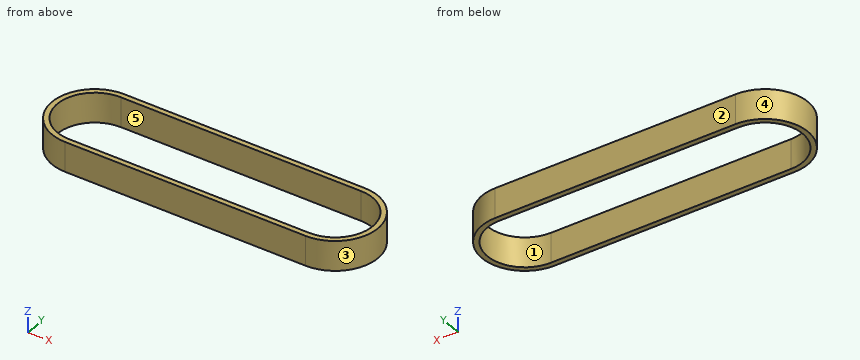
Autodesk Inventor part; units mm, degrees
ref_plane "YZ Plane" through (0, 0, 0) normal (1, 0, 0) x (0, 1, 0)
ref_plane "XZ Plane" through (0, 0, 0) normal (0, 1, 0) x (-1, 0, 0)
ref_plane "XY Plane" through (0, 0, 0) normal (0, 0, 1) x (1, 0, 0)
sketch "Sketch1" plane through (0, 0, 0) normal (0, 0, 1) x (1, 0, 0)
  arc A0 (0, -11.4595) -> (0, 11.4595) centre (0, 0) ccw construction
  arc A1 (-68.9989, 11.4595) -> (-68.9989, -11.4595) centre (-68.9989, 0) ccw construction
  line L0 (0, -11.4595) -> (-68.9989, -11.4595) construction
  line L1 (0, 11.4595) -> (-68.9989, 11.4595) construction
  dimension "Belt_Teeth" = 70
  dimension "Belt_Pitch2" = 3
  dimension "d0" = 22.919
  dimension "d1" = 22.919
  dimension "d2" = 36.0011
  dimension "d3" = 36.0011
  dimension "Center_Distance" = 68.9989
  dimension "d5" = 68.9989
sketch "Sketch2" plane through (0, 0, 0) normal (0, 0, 1) x (1, 0, 0)
  line L0 (35.7235, 34.2567) -> (38.7235, 34.2567)
  point P0 (0, 0)
  dimension "Belt_Pitch2" = 3
sketch "Sketch4" plane through (0, 0, 0) normal (0, 0, 1) x (1, 0, 0)
  line L0 (-16.1422, -21.869) -> (-14.1422, -21.869)
  line L1 (-16.1422, -21.869) -> (-16.1422, -20.349)
  arc A0 (-15.5872, -20.904) -> (-16.1422, -20.349) centre (-16.1422, -20.904) ccw
  line L2 (-15.5872, -20.904) -> (-15.5872, -20.959)
  arc A1 (-15.5872, -20.959) -> (-15.4372, -21.109) centre (-15.4372, -20.959) ccw
  line L3 (-15.4372, -21.109) -> (-14.8472, -21.109)
  line L4 (-14.1422, -21.869) -> (-14.1422, -20.349)
  arc A2 (-14.1422, -20.349) -> (-14.6972, -20.904) centre (-14.1422, -20.904) ccw
  arc A3 (-14.8472, -21.109) -> (-14.6972, -20.959) centre (-14.8472, -20.959) ccw
  line L5 (-14.6972, -20.959) -> (-14.6972, -20.904)
  line L6 (0, 11.4595) -> (-68.9989, 11.4595) construction
  arc A4 (-68.9989, 11.4595) -> (-68.9989, -11.4595) centre (-68.9989, 0) ccw construction
  line L7 (0, -11.4595) -> (-68.9989, -11.4595) construction
  arc A5 (0, -11.4595) -> (0, 11.4595) centre (0, 0) ccw construction
  arc A6 (-68.9989, 12.2195) -> (-68.9989, -12.2195) centre (-68.9989, 0) ccw
  line L8 (-68.9989, 12.2195) -> (0, 12.2195)
  arc A7 (0, -12.2195) -> (0, 12.2195) centre (0, 0) ccw
  line L9 (0, -12.2195) -> (-68.9989, -12.2195)
  arc A8 (-68.9989, 10.6995) -> (-68.9989, -10.6995) centre (-68.9989, 0) ccw
  line L10 (-68.9989, 10.6995) -> (0, 10.6995)
  arc A9 (0, -10.6995) -> (0, 10.6995) centre (0, 0) ccw
  line L11 (0, -10.6995) -> (-68.9989, -10.6995)
  point P0 (-15.1422, -21.109)
  point P1 (-15.1422, -21.869)
  dimension "d9" = 2
  dimension "d10" = 1.52
  dimension "d11" = 0.76
  dimension "d12" = 0.555
  dimension "d13" = 0.555
  dimension "d14" = 0.15
  dimension "d15" = 0.15
  dimension "belt_thickness" = 1.52
  dimension "d44" = 0.76
extrude "Extrusion2" add sketch "Sketch4" along normal mid plane 8.5 contours L8 A7 L9 A6
sketch "Sketch5" plane through (0, 0, 4.25) normal (0, 0, 1) x (1, 0, 0)
  line L0 (-68.9989, 10.6995) -> (0, 10.6995) construction
  arc A0 (0, -10.6995) -> (0, 10.6995) centre (0, 0) ccw construction
  line L1 (0, -10.6995) -> (-68.9989, -10.6995) construction
  arc A1 (-68.9989, 10.6995) -> (-68.9989, -10.6995) centre (-68.9989, 0) ccw construction
  arc A2 (-68.9989, 12.2195) -> (-68.9989, -12.2195) centre (-68.9989, 0) ccw construction
  line L2 (-68.9989, -12.2195) -> (0, -12.2195) construction
  arc A3 (0, -12.2195) -> (0, 12.2195) centre (0, 0) ccw construction
  line L3 (0, 12.2195) -> (-68.9989, 12.2195) construction
  line L4 (-7.7556, -2.6989) -> (-5.7556, -2.6989)
  line L5 (-7.7556, -2.6989) -> (-7.7556, -1.1789) construction
  arc A4 (-7.2006, -1.7339) -> (-7.7556, -1.1789) centre (-7.7556, -1.7339) ccw
  line L6 (-7.2006, -1.7339) -> (-7.2006, -1.7889)
  arc A5 (-7.2006, -1.7889) -> (-7.0506, -1.9389) centre (-7.0506, -1.7889) ccw
  line L7 (-7.0506, -1.9389) -> (-6.4606, -1.9389)
  line L8 (-5.7556, -2.6989) -> (-5.7556, -1.1789)
  arc A6 (-5.7556, -1.1789) -> (-6.3106, -1.7339) centre (-5.7556, -1.7339) ccw
  arc A7 (-6.4606, -1.9389) -> (-6.3106, -1.7889) centre (-6.4606, -1.7889) ccw
  line L9 (-6.3106, -1.7889) -> (-6.3106, -1.7339)
  line L10 (-8.3106, -1.7339) -> (-8.3106, -1.7889)
  arc A8 (-7.7556, -1.1789) -> (-8.3106, -1.7339) centre (-7.7556, -1.7339) ccw
  arc A9 (-8.4606, -1.9389) -> (-8.3106, -1.7889) centre (-8.4606, -1.7889) ccw
  line L11 (-8.4606, -1.9389) -> (-9.0506, -1.9389)
  line L12 (-7.7556, -2.6989) -> (-9.7556, -2.6989)
  line L13 (-9.2006, -1.7889) -> (-9.2006, -1.7339)
  arc A10 (-9.2006, -1.7339) -> (-9.7556, -1.1789) centre (-9.7556, -1.7339) ccw
  line L14 (-9.7556, -2.6989) -> (-9.7556, -1.1789)
  arc A11 (-9.2006, -1.7889) -> (-9.0506, -1.9389) centre (-9.0506, -1.7889) ccw
  line L15 (-17.66, -0.8495) -> (-14.922, -0.8495) construction
  line L16 (-14.922, -0.8495) -> (-14.922, -2.3671) construction
  line L17 (-14.922, -2.3671) -> (-17.66, -2.3671) construction
  line L18 (-17.66, -2.3671) -> (-17.66, -0.8495) construction
  arc A12 (-15.6383, -1.7102) -> (-16.7483, -1.7102) centre (-16.1933, -1.7102) ccw construction
  line L19 (-16.7483, -1.7102) -> (-16.7483, -1.7652) construction
  arc A13 (-16.8983, -1.9152) -> (-16.7483, -1.7652) centre (-16.8983, -1.7652) ccw construction
  line L20 (-16.7483, -1.7102) -> (-16.7483, -1.9152) construction
  line L21 (-15.6383, -1.7102) -> (-15.6383, -1.9152) construction
  point P0 (-6.7556, -1.9389)
  point P1 (-6.7556, -2.6989)
  point P2 (-8.7556, -2.6989)
  point P3 (-8.7556, -1.9389)
  dimension "d22" = 2
  dimension "d23" = 1.52
  dimension "d24" = 0.76
  dimension "d25" = 0.555
  dimension "d26" = 0.555
  dimension "d27" = 0.15
  dimension "d28" = 0.15
  dimension "d29" = 0.76
  dimension "d30" = 1
  dimension "d31" = 2
  dimension "d32" = 0.59
  dimension "d34" = 0.555
  dimension "d35" = 0
  dimension "d36" = 0
  dimension "d37" = 0.15
  dimension "d38" = 0.055
  dimension "d39" = 0.055
  dimension "d40" = 0
  dimension "d41" = 0
  dimension "d42" = 0.205
  dimension "d43" = 0.205
equation "\"Belt_Teeth\" = 70"
equation "\"d13\" = d12"
equation "\"d15\" = d14"
equation "\"d44\" = 0.5 * belt_thickness"
equation "\"d26\" = d25"
equation "\"d28\" = d27"
equation "\"d31\" = d22"
equation "\"d43\" = d42"
equation "\"Belt_Pitch\" = 3"
equation "\"HTD_5mm\" = 5"
equation "\"GT2_3mm\" = 3"
equation "\"Center_Distance_Copy\" = Center_Distance"
properties part number "BELT" material "Rubber"
Read the model definition and answer for the solid it produces. Units are mm, in the model's axes. Face numbers are marked on the shaded views. A direction names the side the tool comes from. Round coordinates to 2 decimals unless told otherwise and drop trailing zeros. Write each loop counter-clockwise with the first axis right and the second up, starting at its lowest first coordinate (ties: lowest second). Pieces come first, ordered by that corner, then holes. Notation, with made-up numbers: M 10.5,62 L 15.5,62 A16 cw 15.5,77 Z; hole C 88.5,-33.5 d10. An arc over 180 degrees is marked long. One line per item, written item: value.
Q1. Which of the six approach directions +Z, -Z, +X, -X, +Y, -Y give full straight-line access (tool end or side, diameter ignored) to the marked faces 4 and 5?
Data:
face 4: +Z, -Z, -X
face 5: +Z, -Z
Q2. For a pull along X with two mould halves and no side action, classify the marked faces 1, 2 and 3 as +X half, -X half, draft (parallel to the pull), parting line (faces both ways), or undercut.
Data:
face 1: undercut
face 2: draft
face 3: +X half
Q3. Find section B-B on x = -11.5. Write down the section's boundary in (y, z), plus the area to 3 significant figures.
Data:
outline: M -12.22,-4.25 L -10.7,-4.25 L -10.7,4.25 L -12.22,4.25 Z; M 10.7,-4.25 L 12.22,-4.25 L 12.22,4.25 L 10.7,4.25 Z
area: 25.8 mm2
Q4. Find section A-A on y = 0. Write down the section's boundary in (x, z).
Data:
outline: M -81.22,-4.25 L -79.7,-4.25 L -79.7,4.25 L -81.22,4.25 Z; M 10.7,-4.25 L 12.22,-4.25 L 12.22,4.25 L 10.7,4.25 Z
Q5. Flat-ended cylindrical pins translate along their axes: pin 1 Ø3 at (x, y) = (-38, -7.5) entering from +Z; pin 2 Ø10 at (x, y) = (-29.5, -6.5) entering from -Z; pin 3 Ø2 at (y, z) = (-6, 2.5) entering from -X; pin 4 Ø3 at (y, z) = (-7, 1) entering from +X. Find the tip coordinate at first contact, or state that the pin passes through.
Data:
pin 1: through
pin 2: z = -4.25
pin 3: x = -80.15
pin 4: x = 10.91
Q6. Find section C-C on z = 2.5. Write down the section's boundary in (x, y), plus the area to 3 significant figures.
Data:
outline: M -69,-12.22 L 0,-12.22 A12.22 ccw 0,12.22 L -69,12.22 A12.22 ccw Z; hole M -69,-10.7 L 0,-10.7 A10.7 ccw 0,10.7 L -69,10.7 A10.7 ccw Z
area: 319 mm2
Q7. Straight lines are drawn through the part: line 1 (Y direction, x = -19, z = -0.75); line 2 (X direction, y = -0.5, z = 0); line 3 (X direction, y = -3, z = -2.5). For each, find the intervals that lie inside material, in ascending order. Write a range as [from, to].
Data:
line 1: [-12.22, -10.7], [10.7, 12.22]
line 2: [-81.21, -79.69], [10.69, 12.21]
line 3: [-80.84, -79.27], [10.27, 11.85]
